Can you work these out from the drawing? Everything is in mm from the part's minimum corner. A direction names the side the tool comes from. Give positions to 0.01 mm unless a question says otherwise; leave off trailing zeros. Write each loop counter-clockwise with the first axis right and the second up, starting at its lowest first coordinate (ties: lowest second). Pieces come first, ordered by that corner, then holes. Notation, with made-up numbers: (58, -37) - (109, -37) arc R26 cw to (109, -14) - close; hole circle Ø5 at (46.25, -24.5). An arc over 180 degrees is marked (long way). Use a Markdown table: item, result.
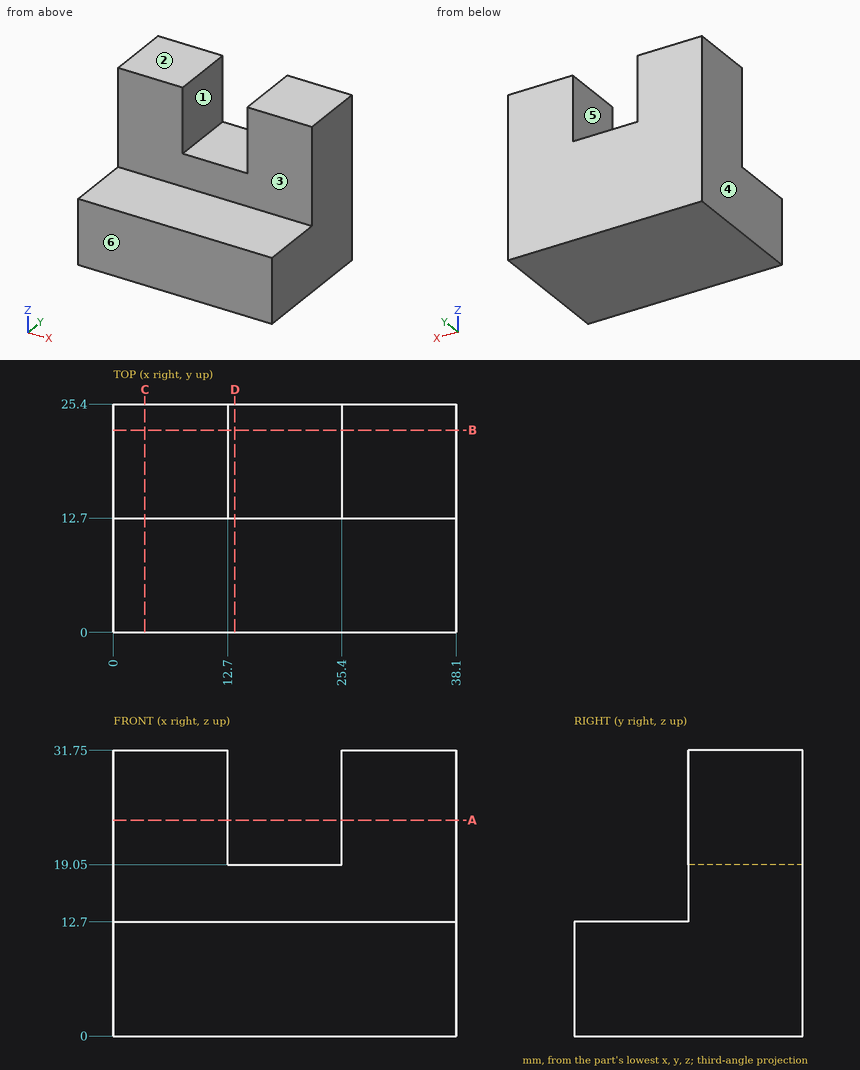
Item 1: If we section it at C-C, the plane x = 3.5: Write out the boundary of the cut face in (y, z).
Values:
| item | result |
|---|---|
| outline | (0, 0) - (25.4, 0) - (25.4, 31.75) - (12.7, 31.75) - (12.7, 12.7) - (0, 12.7) - close |
Item 2: I need wall thicknesses on line 1 along X through (y, z) = (13.25, 20); line 2 along Z through (x, y) = (17.5, 8.5); line 3 along Y through (x, z) = (28, 16). Which ranges of each line are inside material? Lowest first, please. Write a range as [from, to].
Values:
| item | result |
|---|---|
| line 1 | x = [0, 12.7], [25.4, 38.1] |
| line 2 | z = [0, 12.7] |
| line 3 | y = [12.7, 25.4] |
Item 3: If we section it at A-A, the plane z = 24: Write out the boundary of the cut face in (x, y).
Values:
| item | result |
|---|---|
| outline | (0, 12.7) - (12.7, 12.7) - (12.7, 25.4) - (0, 25.4) - close; (25.4, 12.7) - (38.1, 12.7) - (38.1, 25.4) - (25.4, 25.4) - close |
Item 4: Thinking about a two-plate mould opening in X: for the marked faces 4, 5 and 6, which applies, +X half, -X half, draft (parallel to the pull), parting line (faces both ways), or undercut?
Values:
| item | result |
|---|---|
| face 4 | -X half |
| face 5 | undercut |
| face 6 | draft |
Item 5: If we section it at D-D, the plane x = 13.5: Write out the boundary of the cut face in (y, z).
Values:
| item | result |
|---|---|
| outline | (0, 0) - (25.4, 0) - (25.4, 19.05) - (12.7, 19.05) - (12.7, 12.7) - (0, 12.7) - close |
Item 6: Will these pins go through, and if not, where does the flat tip stop? pin 1 Ø1.5 at (x, y) = (18.5, 15) entering from +Z; pin 2 Ø10 at (x, z) = (29, 19) entering from -Y; pin 3 Ø1 at (x, z) = (33.5, 9.5) entering from -Y; pin 4 Ø6.5 at (x, y) = (16.5, 5) entering from +Z.
Values:
| item | result |
|---|---|
| pin 1 | stops at z = 19.05 |
| pin 2 | stops at y = 12.7 |
| pin 3 | stops at y = 0 |
| pin 4 | stops at z = 12.7 |
Item 7: If we section it at B-B, the plane y = 22.5: Write out the boundary of the cut face in (x, z).
Values:
| item | result |
|---|---|
| outline | (0, 0) - (38.1, 0) - (38.1, 31.75) - (25.4, 31.75) - (25.4, 19.05) - (12.7, 19.05) - (12.7, 31.75) - (0, 31.75) - close |
Item 8: For the marked faces 1, 2 and 3, which set-ups out of +Z, -Z, +X, -X, +Y, -Y let a thin tool reach every point of the face, with its end or its side?
Values:
| item | result |
|---|---|
| face 1 | +Z, +Y, -Y |
| face 2 | +Z, +X, -X, +Y, -Y |
| face 3 | +Z, +X, -X, -Y |
